The listing builds one solid part. Answer for the finished solid, in the listing's coordinates (mm). A direction names the side the tool comes from. Round coordinates to 2 decimals unless told otherwise and drop trailing zeros. Write each loop counter-clockwise with the first axis right and the second up, starting at its lowest first coordinate (ties: lowest second). Pieces come first, ordered by that corner, then holes. Notation, with made-up numbers: (24, -14.75) -> (49, -14.75) arc R24 ccw to (49, 16.25) -> close; hole circle Ø6 at (-1.5, -20). An arc over 180 degrees is marked (long way). Write each question's results on one line, items separated by ' | '. Start each with the question number.
```python
from build123d import *

# Parameters (mm, degrees)
SKETCH1_W                     = 104.5
SKETCH1_H                     = 59.5
BOSS_EXTRUDE1_DEPTH           = 73.36
CUT_EXTRUDE2_DEPTH            = 108.944439875
CBORE_FOR_M4_SHCS1_AT_2_COUNT = 2
CBORE_FOR_M4_SHCS1_AT_2_PITCH = 73
CBORE_FOR_M4_SHCS1_AT_3_COUNT = 2
CBORE_FOR_M4_SHCS1_AT_3_PITCH = 83.725742756
CBORE_FOR_M4_SHCS1_AT_4_COUNT = 2
CBORE_FOR_M4_SHCS1_AT_4_PITCH = 41


with BuildPart() as part:
    # Sketch1 → Boss-Extrude1 (new body)
    with BuildSketch(Plane(origin=(0, 0, 0), x_dir=(1, 0, 0), z_dir=(0, 1, 0))):
        Rectangle(SKETCH1_W, SKETCH1_H)
    extrude(amount=BOSS_EXTRUDE1_DEPTH)

    # Sketch6 → Cut-Extrude2 (cut, through all)
    with BuildSketch(Plane.XY.offset(29.75)):
        Polygon((-52.25, 0), (52.25, 73.36), (-52.25, 73.36), align=None)
    extrude(amount=-CUT_EXTRUDE2_DEPTH, mode=Mode.SUBTRACT)

    # Sketch9 → CBORE for M4 SHCS1 (revolve, cut)
    with BuildSketch(Plane(origin=(-1.145450259, -25.214571197, -20.5), x_dir=(0.8184584759172453, 0.5745656822324319, 0), z_dir=(0, 0, 1))):
        Polygon((0, 0), (0, 110.042113793), (2.25, 110.042113793), (2.25, 44), (4, 44), (4, 0.020977491), (4.025, 0), align=None)
    cbore_for_m4_shcs1 = revolve(axis=Axis((2.503041823, -30.411782519, -20.5), (-0.5745656822324319, 0.8184584759172453, 0)), mode=Mode.SUBTRACT)

    # CBORE for M4 SHCS1 at 2: CBORE for M4 SHCS1 ×2
    with Locations(*[Vector(0.8184584759172454, 0.5745656822324319, 0) * (i * CBORE_FOR_M4_SHCS1_AT_2_PITCH) for i in range(1, CBORE_FOR_M4_SHCS1_AT_2_COUNT)]):
        add(cbore_for_m4_shcs1, mode=Mode.SUBTRACT)

    # CBORE for M4 SHCS1 at 3: CBORE for M4 SHCS1 ×2
    with Locations(*[Vector(0.7136093007411902, 0.5009605579174519, 0.48969407317906627) * (i * CBORE_FOR_M4_SHCS1_AT_3_PITCH) for i in range(1, CBORE_FOR_M4_SHCS1_AT_3_COUNT)]):
        add(cbore_for_m4_shcs1, mode=Mode.SUBTRACT)

    # CBORE for M4 SHCS1 at 4: CBORE for M4 SHCS1 ×2
    with Locations(*[(0, 0, i * CBORE_FOR_M4_SHCS1_AT_4_PITCH) for i in range(1, CBORE_FOR_M4_SHCS1_AT_4_COUNT)]):
        add(cbore_for_m4_shcs1, mode=Mode.SUBTRACT)


solid = part.part
```
Q1. For faces 4 (the flat face through (-27.836, 9.808, 22.222)), 5 (the flat face through (22, 20, -29.75)), determine the directions among +Z, -Z, +X, -X, +Y, -Y from which every point of the face is accessible in a straight line to the end or side of a thin tool.
Q2. Determine the mould class of faces 1 (the flat face through (52.25, 36, 0)), 2 (the flat face through (31.91, 51.75, 22.22)), 3 (the flat face through (22, 20, 29.75)) for opening direction X: pulls with the +X half, pulls with the -X half, needs draft (parallel to the pull), parting line crosses it, or undercut.
Q3. The part is cut by section A-A, the plane z = 7.5. Write down the section's boundary in (x, y).
Q4. Find the intervals of material crossed by line 1 (X direction, y = 5, z = -18.5); line 2 (X direction, y = 16, z = 19); line 3 (Y direction, x = -4, z = 17.5), in increasing order.
Q5. The part is cut by section B-B, the plane y = 34. State how many separate pieces and enclosed holes the cut face has, then the cut area to 3 significant figures.
Q6. Each of these flat-tipped pins is pushed along its axis until it touches: pin 1 (1.5 mm diameter, centred on x = 11.5, z = 23, fed in from -Y); pin 2 (3 mm diameter, centred on x = 30, z = 4.5, fed in from +Y); pin 3 (2 mm diameter, centred on x = 6.5, z = 9.5, fed in from +Y); pin 4 (2 mm diameter, centred on x = -12.5, z = -1, fed in from +Y). Where does it stop, or does it pass through?
Q7. The part is cut by section C-C, the plane x = 20. Write down the section's boundary in (y, z).
Answers follow:
1) face 4: none | face 5: -Z, +X, -X, +Y, -Y
2) face 1: pulls with the +X half | face 2: undercut | face 3: needs draft
3) outline: (-52.25, 0) -> (52.25, 0) -> (52.25, 73.36) -> close
4) line 1: -45.13 to -26.59, -18.12 to 52.25 | line 2: -28.03 to 52.25 | line 3: 0 to 33.87
5) separate pieces: 1 | enclosed holes: 2 | area: 3,210 mm^2
6) pin 1: y = 0 | pin 2: y = 58.79 | pin 3: y = 41.95 | pin 4: y = 28.61
7) outline: (0, -29.75) -> (50.72, -29.75) -> (50.72, 29.75) -> (0, 29.75) -> close
